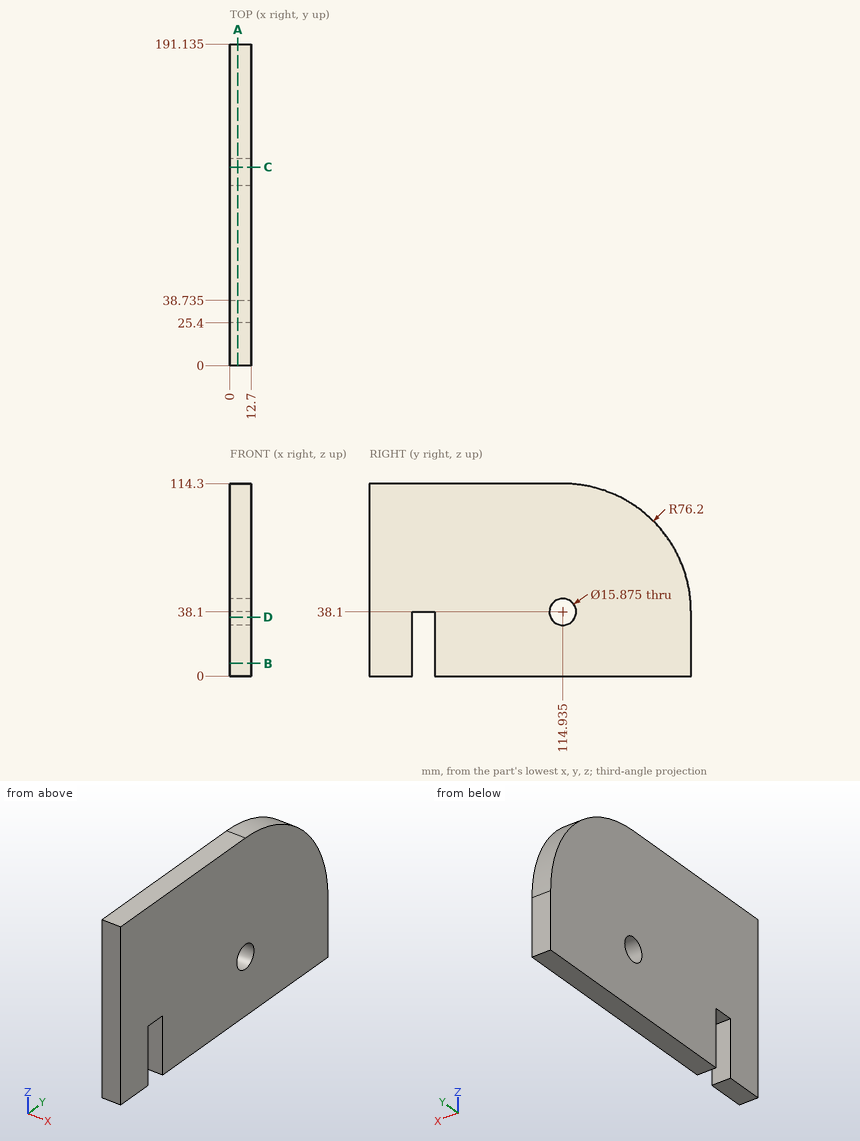
Verification items for this drawing (mm, ordinates from the low corner). Give positions to 0.01 mm unless a question says otherwise; leave off trailing zeros. Loops run counter-clockwise (first coordinate to the right, second up) from the corner with the lowest first, then second, coordinate; pieces in that order, holes last. Notation, with made-up numbers: M 28.25,-33 L 39.25,-33 A21 ccw 39.25,-13 Z; hole C -9.75,38 d11. An arc over 180 degrees is marked long. Write item = value, one per line.
(1) Sectioned sample at A-A, the plane x = 4.75. Record the cut outline in (y, z) (1 decimal), plus the area to 3 significant figures.
Answer below:
outline = M 0,0 L 25.4,0 L 25.4,38.1 L 38.7,38.1 L 38.7,0 L 191.1,0 L 191.1,38.1 A76.2 ccw 114.9,114.3 L 0,114.3 Z; hole C 114.9,38.1 d15.9
area = 19,900 mm2
(2) Sectioned sample at C-C, the plane y = 118. Record the cut outline in (x, z).
Answer below:
outline = M 0,0 L 12.7,0 L 12.7,30.78 L 0,30.78 Z; M 0,45.42 L 12.7,45.42 L 12.7,114.24 L 0,114.24 Z
(3) Material ranges on line 1 (Y direction, x = 11.5, z = 19) (3 decimals); line 2 (Y direction, x = 10.75, z = 34.5) (3 decimals); line 3 (Y direction, x = 10.25, z = 36) (3 decimals), recorded low to high. Write a range as [from, to].
Answer below:
line_1 = [0, 25.4], [38.735, 191.135]
line_2 = [0, 25.4], [38.735, 107.861], [122.009, 191.135]
line_3 = [0, 25.4], [38.735, 107.28], [122.59, 191.135]
(4) Gauge pin test, flat end, axial feed: pin 1 Ø1.5 at (x, z) = (6.5, 78) entering from +Y. Record the tip position at first contact, or that the pin passes through.
Answer below:
pin_1 = 180.31
(5) Sectioned sample at D-D, the plane z = 35. Record the cut outline in (x, y) (3 decimals), plus the area to 3 significant figures.
Answer below:
outline = M 0,0 L 12.7,0 L 12.7,25.4 L 0,25.4 Z; M 0,38.735 L 12.7,38.735 L 12.7,107.628 L 0,107.628 Z; M 0,122.242 L 12.7,122.242 L 12.7,191.135 L 0,191.135 Z
area = 2,070 mm2
(6) Sectioned sample at B-B, the plane z = 7.5. Record the cut outline in (x, y) (3 decimals), plus the area to 3 significant figures.
Answer below:
outline = M 0,0 L 12.7,0 L 12.7,25.4 L 0,25.4 Z; M 0,38.735 L 12.7,38.735 L 12.7,191.135 L 0,191.135 Z
area = 2,260 mm2
